Here's the drawing with two shaded views (mm, measured from the low corner). I have some questions. A direction names the side the tool comes from. Coordinates: 2 decimals unless noted, no trailing zeros. Order: outer loops, then holes, each group sorted by start corner. A loop starts at its lowest first (then second) coordinate and runs counter-clockwise, first axis right, second up. Notation, with made-up numbers: (87, 44.5) -> (108, 44.5) arc R20 cw to (108, 59.5) -> close; hole circle Ø2 at (7.25, -31). An arc over 180 degrees is marked (long way). Write item = value, one per line.
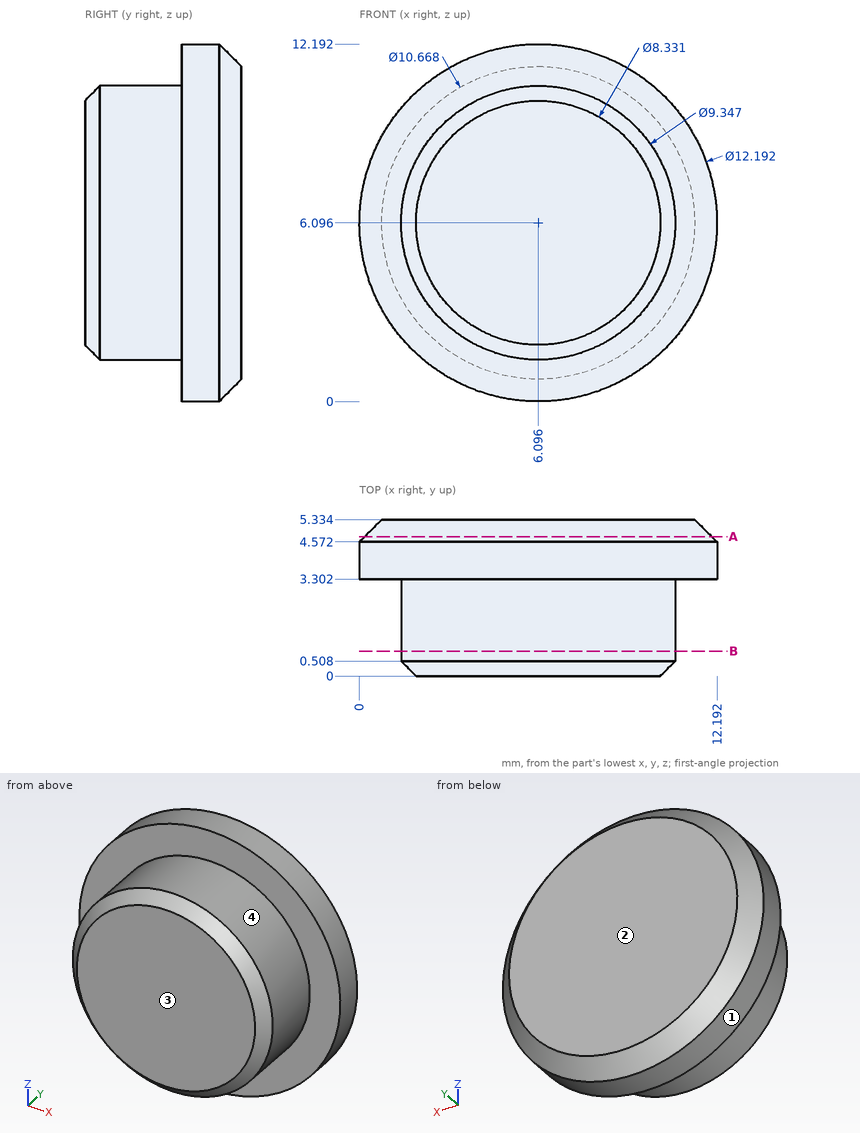
Item 1: I'm going to push a flat-ended pin straight in: P1, Ø1.5, axis at x = 6.5, y = 3.5, coming from the -Z side. Where does the tip first touch, or does it pass through?
A:
P1 = 0
Item 2: If I drill on probe 1 along Y at (x, z) = (1.25, 4.5); probe 2 along Z at (x, y) = (2.5, 1.45); probe 3 along X at (y, z) = (4.95, 9.25) (1 decimal), over which ranges is the centre line in solid material (lowest first)?
A:
probe_1 = 3.3 to 5.33
probe_2 = 3.11 to 9.08
probe_3 = 1.3 to 10.9
Item 3: For the marked faces 3 and 4, which set-ups out of +Z, -Z, +X, -X, +Y, -Y let a thin tool reach every point of the face, with its end or its side?
A:
face_3 = +Z, -Z, +X, -X, -Y
face_4 = -Y
Item 4: I want a section at B-B, the plane y = 0.85. Please give me the cut outline in (x, z), plus the area to 3 significant figures.
A:
outline = circle Ø9.35 at (6.1, 6.1)
area = 68.6 mm2
Item 5: If we mould it in two halves opening along Z, with no side actions, what happens to the marked faces 1 and 2? For each: pulls with the +Z half, pulls with the -Z half, needs draft (parallel to the pull), parting line crosses it, or undercut.
A:
face_1 = parting line crosses it
face_2 = needs draft
Item 6: I want a section at A-A, the plane y = 4.75. Please give me the cut outline in (x, z), plus the area to 3 significant figures.
A:
outline = circle Ø11.84 at (6.1, 6.1)
area = 110 mm2
